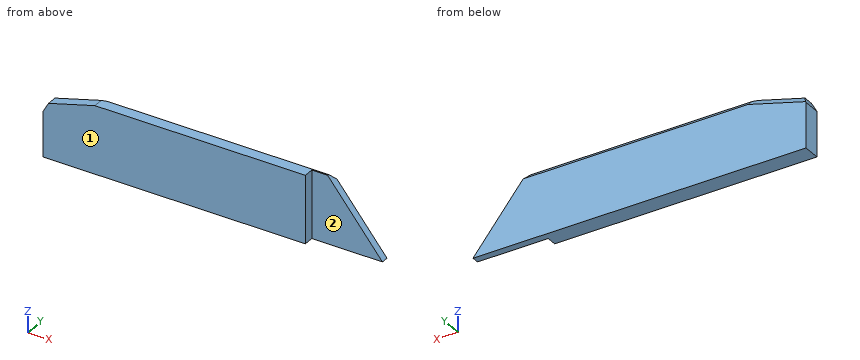
from build123d import *

# Parameters (mm, degrees)
SKETCH1_W           = 91
SKETCH1_H           = 23.5
BOSS_EXTRUDE1_DEPTH = 3.5
BOSS_EXTRUDE2_DEPTH = 2.5
CHAMFER1_SIZE       = 5
CHAMFER1_SIZE2      = 18
CHAMFER2_SIZE       = 2
CHAMFER2_SIZE2      = 2.874083337
CHAMFER3_SIZE       = 2.5
CHAMFER4_SIZE       = 2


with BuildPart() as part:
    # Sketch1 → Boss-Extrude1 (new body)
    with BuildSketch(Plane(origin=(0, 0, 0), x_dir=(1, 0, 0), z_dir=(0, 1, 0))):
        with Locations((4.795180723, 5.722891566)):
            Rectangle(SKETCH1_W, SKETCH1_H)
    extrude(amount=BOSS_EXTRUDE1_DEPTH)

    # Sketch2 → Boss-Extrude2 (add)
    with BuildSketch(Plane(origin=(0, 3.5, 0), x_dir=(1, 0, 0), z_dir=(0, 1, 0))):
        Polygon((-40.704819277, 17.472891566), (-40.704819277, -6.027108434), (55.795180723, -6.027108434), (74.795180723, 17.472891566), align=None)
    extrude(amount=BOSS_EXTRUDE2_DEPTH)

    # Chamfer1
    chamfer1_edges = [part.edges().sort_by_distance(p)[0] for p in [
        (-40.704819277, 3, 6.027108434),
    ]]
    chamfer1_side = [part.faces().sort_by_distance(p)[0] for p in [
        (-40.704819277, 3, -5.722891566),
    ]]
    chamfer(chamfer1_edges, length=CHAMFER1_SIZE, length2=CHAMFER1_SIZE2, reference=chamfer1_side[0])

    # Chamfer2
    chamfer2_edges = [part.edges().sort_by_distance(p)[0] for p in [
        (-40.704819277, 3, 1.027108434),
    ]]
    chamfer2_side = [part.faces().sort_by_distance(p)[0] for p in [
        (-31.704819277, 3, 3.527108434),
    ]]
    chamfer(chamfer2_edges, length=CHAMFER2_SIZE, length2=CHAMFER2_SIZE2, reference=chamfer2_side[0])

    # Chamfer3
    chamfer3_edges = [part.edges().sort_by_distance(p)[0] for p in [
        (-30.741301367, 6, 3.794752298),
    ]]
    chamfer(chamfer3_edges, length=CHAMFER3_SIZE)

    # Chamfer4
    chamfer4_edges = [part.edges().sort_by_distance(p)[0] for p in [
        (21.215566146, 6, 6.027108434),
    ]]
    chamfer(chamfer4_edges, length=CHAMFER4_SIZE)


solid = part.part
The listing builds one solid part. Answer for the finished solid, in the listing's coordinates (mm). Face numbers are marked on the shaded views. A direction names the side the tool comes from. Round coordinates to 2 decimals unless told otherwise and drop trailing zeros. Loops run counter-clockwise (first coordinate to the right, second up) from the corner with the lowest first, then second, coordinate; pieces in that order, holes last. Notation, with made-up numbers: M 11,28.5 L 59,28.5 A18 ccw 59,43.5 Z; hole C 4.25,89.5 d3. An arc over 180 degrees is marked long. Return JSON: item names as keys, results as strings.
Q1. Find section C-C, the plane z = -11.5. Determine the outline of the cut face in (x, y), plus the area to 3 significant figures.
Results list:
{"outline": "M -40.7,0 L 50.3,0 L 50.3,3.5 L 69.97,3.5 L 69.97,6 L -40.7,6 Z", "area": "595 mm2"}
Q2. Find the intervals of material crossed by line 1 along X through (y, z) = (3, -11.75); line 2 along Y through (x, z) = (54, -12); line 3 along X through (y, z) = (5, -2), in increasing order. Write a range as from..to.
Results list:
{"line 1": "x = -40.7..50.3", "line 2": "y = 3.5..6", "line 3": "x = -40.7..62.29"}
Q3. Find section A-A, the plane y = 1.75. Determine the outline of the cut face in (x, z), plus the area to 3 significant figures.
Results list:
{"outline": "M -40.7,-17.47 L 50.3,-17.47 L 50.3,6.03 L -22.7,6.03 L -38.78,1.56 L -40.7,-1.85 Z", "area": "2,090 mm2"}
Q4. Each of these flat-tipped pins is pushed along its axis until it touches: pin 1 Ø2 at (y, z) = (5, -5.5) entering from +X; pin 2 Ø1 at (x, z) = (62.5, 0.5) entering from -Y; pin 3 Ø1.8 at (y, z) = (1.5, -4.5) entering from +X; pin 4 Ø7 at (x, z) = (60.5, -10) entering from -Y. Where does it stop, or does it pass through?
Results list:
{"pin 1": "stops at x = 65.92", "pin 2": "passes through", "pin 3": "stops at x = 50.3", "pin 4": "stops at y = 3.5"}
Q5. Which of the six approach directions +Z, -Z, +X, -X, +Y, -Y give full straight-line access (tool end or side, diameter ignored) to the marked faces 1 and 2?
Results list:
{"face 1": "+Z, -Z, +X, -X, -Y", "face 2": "+Z, -Z, +X, -Y"}
Q6. Find section B-B, the plane x = 54.5. Determine the outline of the cut face in (y, z).
Results list:
{"outline": "M 3.5,-17.47 L 6,-17.47 L 6,4.03 L 4,6.03 L 3.5,6.03 Z"}
